```python
from build123d import *

# Parameters (mm, degrees)
SKETCH1_W      = 65
SKETCH1_H      = 65
EXTRUDE1_DEPTH = 30
SKETCH2_W      = 65
SKETCH2_H      = 5.91
EXTRUDE2_DEPTH = 20
SKETCH3_W      = 50
SKETCH3_H      = 50
EXTRUDE3_DEPTH = 1


with BuildPart() as part:
    # Sketch1 → Extrude1 (new body)
    with BuildSketch(Plane(origin=(0, 0, 0), x_dir=(1, 0, 0), z_dir=(0, 1, 0))):
        Rectangle(SKETCH1_W, SKETCH1_H)
    extrude(amount=EXTRUDE1_DEPTH)

    # Sketch2 → Extrude2 (cut)
    with BuildSketch(Plane(origin=(0, 30, 0), x_dir=(1, 0, 0), z_dir=(0, 1, 0))):
        with Locations((0, 23.635)):
            Rectangle(SKETCH2_W, SKETCH2_H)
        with Locations((0, 11.815)):
            Rectangle(SKETCH2_W, SKETCH2_H)
        with Locations((0, -0.005)):
            Rectangle(SKETCH2_W, SKETCH2_H)
        with Locations((0, -11.825)):
            Rectangle(SKETCH2_W, SKETCH2_H)
        with Locations((0, -23.645)):
            Rectangle(SKETCH2_W, SKETCH2_H)
    extrude(amount=-EXTRUDE2_DEPTH, mode=Mode.SUBTRACT)

    # Sketch3 → Extrude3 (add)
    with BuildSketch(Plane.XZ):
        Rectangle(SKETCH3_W, SKETCH3_H)
    extrude(amount=EXTRUDE3_DEPTH)


solid = part.part
```
Design review of the part built by this model. Coordinates are the model's own, in mm. A direction names the side the tool comes from. Give positions to 0.01 mm unless a question says otherwise; leave off trailing zeros. Loops run counter-clockwise (first coordinate to the right, second up) from the corner with the lowest first, then second, coordinate; pieces in that order, holes last. Notation, with made-up numbers: (48, 14.25) -> (72, 14.25) arc R14 ccw to (72, 18.25) -> close; hole circle Ø5 at (35.25, -15). An arc over 180 degrees is marked (long way). One line per item, written item: value.
Q1. Draft analysis for pull direction Z (two halves, no side actions). For faces 1 (the flat face through (0, 20, 2.96)), 2 (the flat face through (32.5, 8, 0)), 3 (the flat face through (0, 15, 32.5)), state which applies: pulls with the +Z half, pulls with the -Z half, needs draft (parallel to the pull), parting line crosses it, or undercut.
Numbers:
face 1: undercut
face 2: needs draft
face 3: pulls with the +Z half
Q2. We need section C-C on z = -1. Give the boundary of the cut face in (x, y), and give its area (3 significant figures).
Numbers:
outline: (-32.5, 0) -> (-25, 0) -> (-25, -1) -> (25, -1) -> (25, 0) -> (32.5, 0) -> (32.5, 10) -> (-32.5, 10) -> close
area: 700 mm^2
Q3. Machinability: for faces 4 (the flat face through (0, 20, -20.68)), 5 (the flat face through (0, 30, -30)), which of the approach directions +Z, -Z, +X, -X, +Y, -Y give a long, thin tool a straight path to every point of the face, cutting with its end or side? Answer none if there is none.
Numbers:
face 4: +X, -X, +Y
face 5: +Z, -Z, +X, -X, +Y
Q4. We need section B-B on x = 22.5. Give the boundary of the cut face in (y, z).
Numbers:
outline: (-1, -25) -> (0, -25) -> (0, -32.5) -> (30, -32.5) -> (30, -26.59) -> (10, -26.59) -> (10, -20.68) -> (30, -20.68) -> (30, -14.77) -> (10, -14.77) -> (10, -8.86) -> (30, -8.86) -> (30, -2.95) -> (10, -2.95) -> (10, 2.96) -> (30, 2.96) -> (30, 8.87) -> (10, 8.87) -> (10, 14.78) -> (30, 14.78) -> (30, 20.69) -> (10, 20.69) -> (10, 26.6) -> (30, 26.6) -> (30, 32.5) -> (0, 32.5) -> (0, 25) -> (-1, 25) -> close
Q5. We need section A-A on y = 16. Give the boundary of the cut face in (x, z), and give its area (3 significant figures).
Numbers:
outline: (-32.5, -32.5) -> (32.5, -32.5) -> (32.5, -26.59) -> (-32.5, -26.59) -> close; (-32.5, -20.68) -> (32.5, -20.68) -> (32.5, -14.77) -> (-32.5, -14.77) -> close; (-32.5, -8.86) -> (32.5, -8.86) -> (32.5, -2.95) -> (-32.5, -2.95) -> close; (-32.5, 2.96) -> (32.5, 2.96) -> (32.5, 8.87) -> (-32.5, 8.87) -> close; (-32.5, 14.78) -> (32.5, 14.78) -> (32.5, 20.69) -> (-32.5, 20.69) -> close; (-32.5, 26.6) -> (32.5, 26.6) -> (32.5, 32.5) -> (-32.5, 32.5) -> close
area: 2,300 mm^2
Q6. For L1, parallel to Z at x = -14.5, y = 17; L2, parallel to Y at x = -27.5, z = -11; L3, parallel to Y at x = 26, z = 29.5, list the stretches that pass through material, from the lowest coordinate up.
Numbers:
L1: z = -32.5 to -26.59, -20.68 to -14.77, -8.86 to -2.95, 2.96 to 8.87, 14.78 to 20.69, 26.6 to 32.5
L2: y = 0 to 10
L3: y = 0 to 30
Q7. For pin 1 Ø4.5 at (x, z) = (-11, -1) entering from +Y; pin 2 Ø0.8 at (y, z) = (-0.5, -6.5) entering from +X; pin 3 Ø3 at (x, z) = (7.5, -24.5) entering from +Y, all flat-tipped, find the tip position at first contact; note any pin that passes through.
Numbers:
pin 1: stops at y = 30
pin 2: stops at x = 25
pin 3: stops at y = 10
